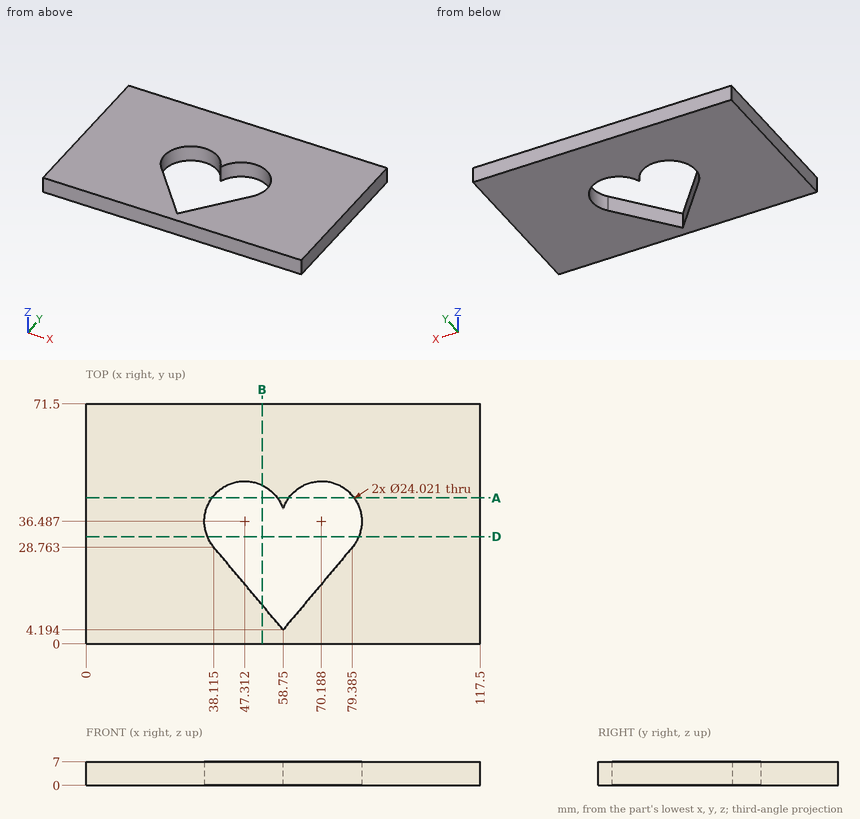
The drawing under review shows one solid part. Ordinate dimensions are in mm from its lowest x, y, z. Coordinates: 2 decimals unless noted, no trailing zeros. Order: outer loops, then holes, each group sorted by start corner. A loop starts at its lowest first (then second) coordinate and runs counter-clockwise, first axis right, second up. Notation, with made-up numbers: M 33.25,13 L 65.25,13 A22 cw 65.25,28 Z; hole C -4,-16 d11. An arc over 180 degrees is marked long. Use a Markdown table: item, result.
(1) For P1, Ø21.5, axis at x = 47.31, y = 36.49, coming from the +Z side, flat-tipped, find the tip position at first contact; note if it passes through.
Worked answers:
| item | result |
|---|---|
| P1 | passes through |
(2) Add section B-B (x = 52.5). Give the boundary of the cut face in (y, z) (1 decimal), then the cut area to 3 significant figures.
Worked answers:
| item | result |
|---|---|
| outline | M 0,0 L 11.6,0 L 11.6,7 L 0,7 Z; M 47.3,0 L 71.5,0 L 71.5,7 L 47.3,7 Z |
| area | 251 mm2 |
(3) Add section D-D (y = 32). Give the boundary of the cut face in (x, z).
Worked answers:
| item | result |
|---|---|
| outline | M 0,0 L 36.17,0 L 36.17,7 L 0,7 Z; M 81.33,0 L 117.5,0 L 117.5,7 L 81.33,7 Z |
(4) Wall thickness on probe 1 along X at (y, z) = (43.5, 1.25) (1 decimal); probe 2 along X at (y, z) = (47.5, 1.25) (1 decimal); probe 3 along Y at (x, z) = (61, 6.5) (1 decimal): over which ranges is each line inside the solid? List them lowest first.
Worked answers:
| item | result |
|---|---|
| probe 1 | x = 0 to 37.6, 57.1 to 60.4, 79.9 to 117.5 |
| probe 2 | x = 0 to 42.5, 52.1 to 65.4, 75 to 117.5 |
| probe 3 | y = 0 to 6.9, 44.2 to 71.5 |
(5) Add section A-A (y = 43.5). Give the boundary of the cut face in (x, z).
Worked answers:
| item | result |
|---|---|
| outline | M 0,0 L 37.56,0 L 37.56,7 L 0,7 Z; M 57.06,0 L 60.44,0 L 60.44,7 L 57.06,7 Z; M 79.94,0 L 117.5,0 L 117.5,7 L 79.94,7 Z |
